```python
from build123d import *

# Parameters (mm, degrees)
F1_DEPTH = 30
F2_R     = 4
F3_DEPTH = 25
F5_DEPTH = 25
F6_R     = 10
F7_D     = 8


with BuildPart() as f1:
    # F0 (on Right) → F1 (new body, symmetric)
    with BuildSketch(Plane.YZ):
        Polygon((-89.018595, 22.871135), (-105.332031, -24.392718), (-146.828609, -10.51621), (-150, -20), (-130, -90), (-81.489667, -90), (-29.716161, 60), (-24.538811, 75), (-19.36146, 90), (-80, 90), (-127.665719, 46.788867), (-130.83711, 37.305077), align=None)
        Polygon((150, 90), (-19.36146, 90), (-24.538811, 75), (-29.716161, 60), (150, 60), align=None)
    extrude(amount=F1_DEPTH, both=True)

    # F2 (on face) → F3 (join)
    with BuildSketch(Plane.YZ.offset(30)):
        Polygon((-80, 90), (-127.665719, 46.788867), (-150, -20), (-130, -90), (150, -90), (150, 90), align=None)
        with Locations((-121.254994, -3.25178)):
            Circle(F2_R, mode=Mode.SUBTRACT)
        with BuildLine():
            Line((71, -53), (36, -53))
            ThreePointArc((36, -53), (33, -50), (36, -47))
            Line((36, -47), (71, -47))
            ThreePointArc((71, -47), (74, -50), (71, -53))
        make_face(mode=Mode.SUBTRACT)
        with Locations((-114.753178, 15.885422)):
            Circle(F2_R, mode=Mode.SUBTRACT)
        with BuildLine():
            Line((103, 50), (103, 15))
            ThreePointArc((103, 15), (100, 12), (97, 15))
            Line((97, 15), (97, 50))
            ThreePointArc((97, 50), (100, 53), (103, 50))
        make_face(mode=Mode.SUBTRACT)
    extrude(amount=F3_DEPTH)

    # F4 (on face) → F5 (join)
    with BuildSketch(Plane(origin=(-30, 0, 0), x_dir=(0, -1, 0), z_dir=(-1, 0, 0))):
        Polygon((29.716161, 60), (-150, 60), (-150, -90), (81.489667, -90), align=None)
        with BuildLine():
            Line((-71, -47), (-36, -47))
            ThreePointArc((-36, -47), (-33, -50), (-36, -53))
            Line((-36, -53), (-71, -53))
            ThreePointArc((-71, -53), (-74, -50), (-71, -47))
        make_face(mode=Mode.SUBTRACT)
        with BuildLine():
            ThreePointArc((-97, 15), (-100, 12), (-103, 15))
            Line((-103, 15), (-103, 50))
            ThreePointArc((-103, 50), (-100, 53), (-97, 50))
            Line((-97, 50), (-97, 15))
        make_face(mode=Mode.SUBTRACT)
        Polygon((130.83711, 37.305077), (127.665719, 46.788867), (80, 90), (-150, 90), (-150, 60), (29.716161, 60), (81.489667, -90), (130, -90), (150, -20), (146.828609, -10.51621), (105.332031, -24.392718), (89.018595, 22.871135), align=None)
        Polygon((146.828609, -10.51621), (130.83711, 37.305077), (89.018595, 22.871135), (105.332031, -24.392718), align=None)
    extrude(amount=F5_DEPTH)

    # F6
    f6_edges = [f1.edges().sort_by_distance(p)[0] for p in [
        (55, 35, 90),
        (55, -103.832859, 68.394433),
        (55, -140, -55),
        (-55, -140, -55),
        (-55, -103.832859, 68.394433),
        (-55, 35, 90),
        (0, 150, 90),
        (-42.5, 150, -90),
        (42.5, 150, -90),
        (-55, -138.832859, 13.394433),
        (55, -138.832859, 13.394433),
    ]]
    fillet(f6_edges, radius=F6_R)

    # F7 (through all)
    with Locations(Plane.YZ.offset(30)):
        with Locations((-114.753178, 15.885422), (-121.254994, -3.25178)):
            Hole(F7_D / 2)


solid = f1.part
```
For this review, take the finished solid that the model builds, in its own axes (mm). A direction names the side the tool comes from. Give positions to 0.01 mm unless a question says otherwise; leave off trailing zeros. Write each loop counter-clockwise with the first axis right and the second up, starting at its lowest first coordinate (ties: lowest second). Pieces come first, ordered by that corner, then holes. Notation, with made-up numbers: M 31.5,25.5 L 39.5,25.5 A5 ccw 39.5,33.5 Z; hole C -4.75,0 d8. An arc over 180 degrees is marked long. Answer as CSV lines item,"result".
1. Wall thickness on line 1 (X direction, y = 130, z = 49); line 2 (Z direction, x = -25, y = 132.5); line 3 (Z direction, x = -45, y = 39.5): over which ranges is each line inside the solid? List them lowest first.
Findings:
line 1,"x = -55 to -30, 30 to 55"
line 2,"z = 60 to 90"
line 3,"z = -90 to -53, -47 to 90"
2. Draft analysis for pull direction Z (two halves, no side actions). For faces 4 (the cylindrical face through (42, 33, -50)), 5 (the flat face through (-55, 7, -4)), 6 (the cylindrical face through (42.68, 146.99, -87.15)), state which applies: +Z half, -Z half, draft (parallel to the pull), parting line (faces both ways), or undercut.
Findings:
face 4,"undercut"
face 5,"draft"
face 6,"-Z half"
3. For pin 1 (12 mm diameter, centred on x = 10, z = -23, fed in from +Y); pin 2 (20 mm diameter, centred on x = 42, z = 29.5, fed in from -Y); pin 3 (18 mm diameter, centred on x = 3, y = 60, fed in from -Z), all flat-tipped, find the tip position at first contact; note any pin that passes through.
Findings:
pin 1,"stops at y = -56.29"
pin 2,"stops at y = -136.79"
pin 3,"stops at z = 60"
4. For faces 1 (the flat face through (30, 58, -14)), 2 (the cylindrical face through (42, 100, 12)), 3 (the cylindrical face through (52.148, -136.137, 11.973)), list the 3-axis set-ups (+Z, -Z, +X, -X, +Y, -Y) from which the entire face can be reached by the end or side of a thin tool; tool diameter is ignored.
Findings:
face 1,"-Z, +Y"
face 2,"+X, -X"
face 3,"+Z, +X, -Y"
5. Consider section C-C, the plane x = -7.5. Write out the cut boundary in (y, z).
Findings:
outline,"M -150,-20 L -130,-90 L -81.49,-90 L -29.72,60 L 150,60 L 150,80 A10 ccw 140,90 L -80,90 L -127.67,46.79 L -130.84,37.31 L -89.02,22.87 L -105.33,-24.39 L -146.83,-10.52 Z"
6. Consider section B-B, the plane y = 13.5. Write out the cut boundary in (x, z), then the cut area to 3 significant figures.
Findings:
outline,"M -55,-90 L -30,-90 L -30,60 L 30,60 L 30,-90 L 55,-90 L 55,80 A10 ccw 45,90 L -45,90 A10 ccw -55,80 Z"
area,"10,800 mm2"
7. Consider section A-A, the plane y = 100. Write out the cut boundary in (x, z).
Findings:
outline,"M -55,-90 L -30,-90 L -30,12 L -55,12 Z; M -55,53 L -30,53 L -30,60 L 30,60 L 30,53 L 55,53 L 55,80 A10 ccw 45,90 L -45,90 A10 ccw -55,80 Z; M 30,-90 L 55,-90 L 55,12 L 30,12 Z"
8. Consider section D-D, the plane x = 37. Write out the cut boundary in (y, z) (3 decimals), then the cut area to 3 significant figures.
Findings:
outline,"M -150,-20 L -130,-90 L 140,-90 A10 ccw 150,-80 L 150,80 A10 ccw 140,90 L -80,90 L -127.666,46.789 Z; hole C -121.255,-3.252 d8; hole C -114.753,15.885 d8; hole M 36,-53 L 71,-53 A3 ccw 71,-47 L 36,-47 A3 ccw Z; hole M 97,15 A3 ccw 103,15 L 103,50 A3 ccw 97,50 Z"
area,"49,900 mm2"
